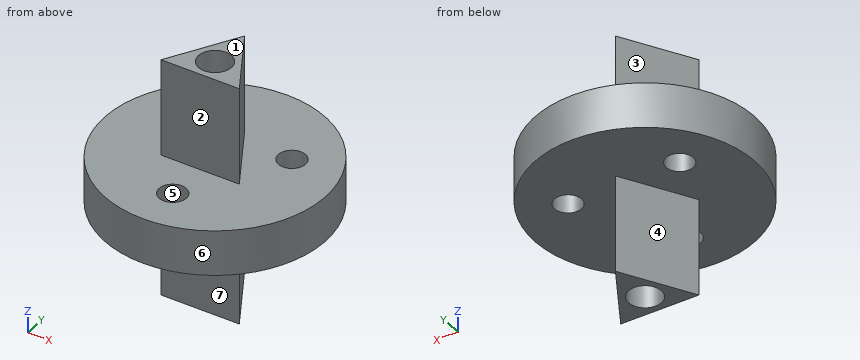
```python
from build123d import *

# Parameters (mm, degrees)
SKETCH3_R                = 17
SKETCH3_R_2              = 2.1
BOSS_EXTRUDE1_DEPTH      = 7
SKETCH4_R                = 2.55
BOSS_EXTRUDE2_DEPTH      = 15
BOSS_EXTRUDE2_DEPTH_BACK = 22
SKETCH9_R                = 2.55
CUT_EXTRUDE1_DEPTH       = 23


with BuildPart() as part:
    # Sketch3 → Boss-Extrude1 (new body)
    with BuildSketch(Plane.XY):
        Circle(SKETCH3_R)
        with Locations((8.660254038, 5)):
            Circle(SKETCH3_R_2, mode=Mode.SUBTRACT)
        with Locations((0, -10)):
            Circle(SKETCH3_R_2, mode=Mode.SUBTRACT)
        with Locations((-8.660254038, 5)):
            Circle(SKETCH3_R_2, mode=Mode.SUBTRACT)
    extrude(amount=BOSS_EXTRUDE1_DEPTH)

    # Sketch4 → Boss-Extrude2 (add, two sides)
    with BuildSketch(Plane.XY.offset(7)) as boss_extrude2_sk:
        Polygon((0, 7), (6.062177826, -3.5), (-6.062177826, -3.5), align=None)
        Circle(SKETCH4_R, mode=Mode.SUBTRACT)
    extrude(amount=BOSS_EXTRUDE2_DEPTH)
    extrude(boss_extrude2_sk.sketch, amount=-BOSS_EXTRUDE2_DEPTH_BACK)

    # Sketch9 → Cut-Extrude1 (cut, through all)
    with BuildSketch(Plane.XY.offset(7)):
        Circle(SKETCH9_R)
    extrude(amount=-CUT_EXTRUDE1_DEPTH, mode=Mode.SUBTRACT)


solid = part.part
```
Could you check a few things on this model? Use its own coordinates, in mm. Face numbers are marked on the shaded views. A direction names the side the tool comes from. Coordinates: 2 decimals unless noted, no trailing zeros. Order: outer loops, then holes, each group sorted by start corner. A loop starts at its lowest first (then second) coordinate and runs counter-clockwise, first axis right, second up. Notation, with made-up numbers: M -8,53 L 25,53 A18 ccw 25,62 Z; hole C 67.25,28.25 d8. An arc over 180 degrees is marked long. Use one line per item in the form item = value. Start each with the question number.
1. Suppose I cut it at A-A on y = 0.5. Write out the boundary of the cut face in (x, z), then the cut area to 3 significant figures.
2. Suppose I cut it at D-D on z = 5.5. Write out the boundary of the cut face in (x, y), then the cut area to 3 significant figures.
3. We'd pull the mould along X, two halves only. Please class the marked faces 4, 5, 6 and 7: +X half, -X half, draft (parallel to the pull), parting line (faces both ways), or undercut.
4. Suppose I cut it at C-C on y = 5. Write out the boundary of the cut face in (x, z).
5. On a 3-axis mill with a long thin cutter (end or side, diameter ignored), from which of +Z, -Z, +X, -X, +Y, -Y can I reach the whole of each face in a straight line? I mean the marked faces 1, 2 and 3. Say none if no direction works.
6. Suppose I cut it at B-B on x = -1. Write out the boundary of the cut face in (y, z), then the cut area to 3 significant figures.
7. Please list where these lines run through material, in increasing order: line 1 (Z direction, x = 3.5, y = 6); line 2 (X direction, y = 2, z = 15); line 3 (Y direction, x = -0.5, z = 11).
8. For pin 1 (3.5 mm diameter, centred on x = 0, y = -10, fed in from -Z); pin 2 (6.5 mm diameter, centred on x = 8.66, y = 5, fed in from +Z); pin 3 (10 mm diameter, centred on x = -4.5, z = 14, fed in from +Y); pin 4 (10 mm diameter, centred on x = -0.5, z = 10, fed in from +Y), each with a flat end and sliding along its axis, tell me the tip position at first contact or that it passes through.
Geometry says:
q1.outline = M -16.99,0 L -3.75,0 L -3.75,-15 L -2.5,-15 L -2.5,22 L -3.75,22 L -3.75,7 L -16.99,7 Z; M 2.5,-15 L 3.75,-15 L 3.75,0 L 16.99,0 L 16.99,7 L 3.75,7 L 3.75,22 L 2.5,22 Z
q1.area = 278 mm^2
q2.outline = C 0,0 d34; hole C -8.66,5 d4.2; hole C 0,0 d5.1; hole C 0,-10 d4.2; hole C 8.66,5 d4.2
q2.area = 846 mm^2
q3.face_4 = -X half
q3.face_5 = undercut
q3.face_6 = parting line
q3.face_7 = draft
q4.outline = M -16.25,0 L -10.76,0 L -10.76,7 L -16.25,7 Z; M -6.56,0 L -1.15,0 L -1.15,-15 L 1.15,-15 L 1.15,0 L 6.56,0 L 6.56,7 L 1.15,7 L 1.15,22 L -1.15,22 L -1.15,7 L -6.56,7 Z; M 10.76,0 L 16.25,0 L 16.25,7 L 10.76,7 Z
q5.face_1 = +Z, +X, -X, +Y, -Y
q5.face_2 = +Z, +X, -X, -Y
q5.face_3 = +Z, -X, +Y
q6.outline = M -16.97,0 L -11.85,0 L -11.85,7 L -16.97,7 Z; M -8.15,0 L -3.5,0 L -3.5,-15 L -2.35,-15 L -2.35,22 L -3.5,22 L -3.5,7 L -8.15,7 Z; M 2.35,-15 L 5.27,-15 L 5.27,0 L 16.97,0 L 16.97,7 L 5.27,7 L 5.27,22 L 2.35,22 Z
q6.area = 301 mm^2
q7.line_1 = 0 to 7
q7.line_2 = -2.89 to -1.58, 1.58 to 2.89
q7.line_3 = -3.5 to -2.5, 2.5 to 6.13
q8.pin_1 = through
q8.pin_2 = 7
q8.pin_3 = 7
q8.pin_4 = 17
